from build123d import *

# Parameters (mm, degrees)
PAD_DEPTH    = 1219.2
SKETCH001_R  = 3
PAD001_DEPTH = 2.54
SKETCH002_R  = 5
PAD002_DEPTH = 2
FILLET_R     = 2


with BuildPart() as part:
    # Sketch → Pad (new body)
    with BuildSketch(Plane.XZ):
        Polygon((0, 0), (0, 16.51), (7.952592, 29.21), (0, 29.21), (0, 50.8), (2.54, 50.8), (2.54, 31.75), (12.54, 31.75), (2.54, 15.780364), (2.54, 0), align=None)
    extrude(amount=PAD_DEPTH)

    # Sketch001 (on Face4 of Pad) → Pad001 (join)
    with BuildSketch(Plane(origin=(0, 0, 0), x_dir=(0, 0, -1), z_dir=(-1, 0, 0))):
        with Locations((-44.45, 12.7)):
            Circle(SKETCH001_R)
        with Locations((-6.35, 12.7)):
            Circle(SKETCH001_R)
        with Locations((-44.45, 1206.5)):
            Circle(SKETCH001_R)
        with Locations((-6.35, 1206.5)):
            Circle(SKETCH001_R)
    extrude(amount=PAD001_DEPTH)

    # Sketch002 (on Face20 of Pad001) → Pad002 (join)
    with BuildSketch(Plane(origin=(-2.54, 0, 0), x_dir=(0, 0, -1), z_dir=(-1, 0, 0))):
        with Locations((-44.45, 12.7)):
            Circle(SKETCH002_R)
        with Locations((-6.35, 12.7)):
            Circle(SKETCH002_R)
        with Locations((-44.45, 1206.5)):
            Circle(SKETCH002_R)
        with Locations((-6.35, 1206.5)):
            Circle(SKETCH002_R)
    extrude(amount=PAD002_DEPTH)

    # Fillet
    fillet_edges = [part.edges().sort_by_distance(p)[0] for p in [
        (12.54, -609.6, 31.75),
        (0, -609.6, 29.21),
        (0, -609.6, 16.51),
        (7.952592, -609.6, 29.21),
    ]]
    fillet(fillet_edges, radius=FILLET_R)


solid = part.part
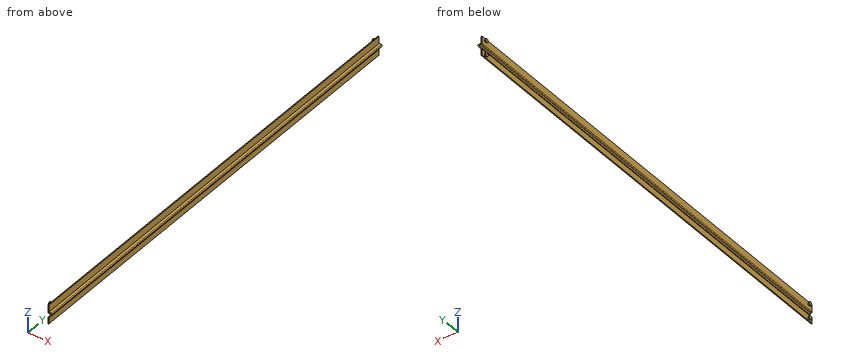
Geometry: final body of the model. Coordinates: model frame, mm. Give positions to 0.01 mm unless a question says otherwise; leave off trailing zeros. Write each loop counter-clockwise with the first axis right and the second up, starting at its lowest first coordinate (ties: lowest second). Pieces come first, ordered by that corner, then holes. Notation, with made-up numbers: (-37.75, 19.25) -> (-13.75, 19.25) arc R34 cw to (-13.75, 52.25) -> close; hole circle Ø4 at (14, -5). An arc over 180 degrees is marked (long way). Answer as a JSON object with one key per item and string values.
1. Cut plane A-A on y = -620. Output: boundary loops of the cut face in (x, z).
Ans:
{"outline": "(0, 0) -> (2.54, 0) -> (2.54, 15.78) -> (10.62, 28.69) arc R2 ccw to (8.93, 31.75) -> (2.54, 31.75) -> (2.54, 50.8) -> (0, 50.8) -> (0, 31.21) arc R2 ccw to (2, 29.21) -> (4.34, 29.21) arc R2 cw to (6.04, 26.15) -> (0.3, 17) arc R2 ccw to (0, 15.94) -> close"}
2. Ray query, probe 1 along X at (y, z) = (-238, 22); probe 2 along X at (y, z) = (-1014, 38.5); probe 3 along Z at (x, y) = (1, -721). Return the intervals inside material, ascending. Write a range as from..to.
Ans:
{"probe 1": "x = 3.44..6.43", "probe 2": "x = 0..2.54", "probe 3": "z = 0..18.11, 29.48..50.8"}
3. Contact query for flat-ended pins moving along their axis: pin 1 (1 mm diameter, centred on x = 2, z = 21.5, fed in from -Y); pin 2 (10 mm diameter, centred on y = -621, z = 38, fed in from -X); pin 3 (4 mm diameter, centred on x = 4.5, y = -201.5, fed in from +Z); pin 4 (5 mm diameter, centred on y = -1206, z = 5, fed in from +X). Output: stop coordinate, or through.
Ans:
{"pin 1": "passes through", "pin 2": "stops at x = 0", "pin 3": "stops at z = 50.8", "pin 4": "stops at x = 2.54"}
